Can you work these out from the model? Positions are in its coordinate system, mm. A direction names the side the tool comes from. Give positions to 0.01 mm unless a question says otherwise; leave off trailing zeros. Loops run counter-clockwise (first coordinate to the right, second up) from the corner with the lowest first, then second, coordinate; pieces in that order, holes last. Notation, with made-up numbers: (52, 65.5) -> (57, 65.5) arc R20 cw to (57, 86.5) -> close; hole circle Ø2 at (82, 75.5). An arc over 180 degrees is marked (long way). One line per question, with ' | ' between items.
from build123d import *

# Parameters (mm, degrees)
SKETCH_1_R      = 2.25
SKETCH_1_R_2    = 2.5
SKETCH_1_R_3    = 4
EXTRUDE_1_DEPTH = 2


with BuildPart() as part:
    # 草图1 → 凸台-拉伸1 (new body)
    with BuildSketch(Plane.XY):
        with BuildLine():
            Line((-97.333495067, -2.569668399), (0.921282848, -2.569581138))
            Line((0.921282848, -2.569581138), (99.176060763, -2.569468011))
            ThreePointArc((99.176060763, -2.569468011), (102.832215453, -3.990464351), (105.660516847, -6.708443184))
            ThreePointArc((105.660516847, -6.708443184), (128.420905518, 0.379743237), (105.718891057, 7.652721898))
            ThreePointArc((105.718891057, 7.652721898), (102.151642887, 4.54858247), (97.556982938, 3.430530125))
            Line((97.556982938, 3.430530125), (0.92127673, 3.430418862))
            Line((0.92127673, 3.430418862), (-95.714429479, 3.430333039))
            ThreePointArc((-95.714429479, 3.430333039), (-100.309091708, 4.548376014), (-103.876346209, 7.652508166))
            ThreePointArc((-103.876346209, 7.652508166), (-126.578345836, 0.379483205), (-103.81794271, -6.708656797))
            ThreePointArc((-103.81794271, -6.708656797), (-100.989646859, -3.990672195), (-97.333495067, -2.569668399))
        make_face()
        with Locations((-119.735572513, -5.226431967)):
            Circle(SKETCH_1_R, mode=Mode.SUBTRACT)
        with Locations((-121.081680504, 2.30686036)):
            Circle(SKETCH_1_R_2, mode=Mode.SUBTRACT)
        with Locations((-108.9521941, 5.556946446)):
            Circle(SKETCH_1_R_2, mode=Mode.SUBTRACT)
        with Locations((-112.202280186, -6.572539958)):
            Circle(SKETCH_1_R_2, mode=Mode.SUBTRACT)
        with Locations((-114.078604371, 0.43031673)):
            Circle(SKETCH_1_R_3, mode=Mode.SUBTRACT)
        with Locations((115.921163949, 0.430551269)):
            Circle(SKETCH_1_R_3, mode=Mode.SUBTRACT)
        with Locations((110.794757573, 5.556946446)):
            Circle(SKETCH_1_R_2, mode=Mode.SUBTRACT)
        with Locations((122.924243977, 2.30686036)):
            Circle(SKETCH_1_R_2, mode=Mode.SUBTRACT)
        with Locations((121.578135986, -5.226431967)):
            Circle(SKETCH_1_R, mode=Mode.SUBTRACT)
        with Locations((114.04484366, -6.572539958)):
            Circle(SKETCH_1_R_2, mode=Mode.SUBTRACT)
    extrude(amount=EXTRUDE_1_DEPTH)


solid = part.part
Q1. If we section it at B-B (x = 72): Write out the boundary of the cut face in (y, z).
Entries:
outline: (-2.57, 0) -> (3.43, 0) -> (3.43, 2) -> (-2.57, 2) -> close
Q2. For pin 1 Ø4.5 at (x, y) = (114.04, -6.57) entering from -Z; pin 2 Ø0.6 at (x, z) = (28.5, 1) entering from -Y; pin 3 Ø1 at (y, z) = (10, 1) entering from -X; pin 4 Ø1 at (x, z) = (30, 0.5) entering from +Y, each with a flat end and sliding along its axis, tell me the tip position at first contact or that it passes through.
Entries:
pin 1: through | pin 2: y = -2.57 | pin 3: x = -122.68 | pin 4: y = 3.43
Q3. If we mould it in two halves opening along X, with no side actions, what happens to faces 1 (the face through (116.43, -5.82, 0.99)), 2 (the face through (-1, 1, 0))? For each: pulls with the +X half, pulls with the -X half, needs draft (parallel to the pull), parting line crosses it, or undercut.
Entries:
face 1: undercut | face 2: needs draft
Q4. If I drill on probe 1 along X at (y, z) = (-5.5, 0.2); probe 2 along X at (y, z) = (-3.25, 0.8); probe 3 along X at (y, z) = (7.25, 0.8), over which ranges is the centre line in solid material (lowest first)? Write a range as from..to.
Entries:
probe 1: -125.08..-121.97, -117.5..-114.46, -109.94..-102.83, 104.67..111.79, 116.3..119.34, 123.81..126.92 | probe 2: -126.02..-120.81, -118.66..-115.65, -112.51..-99.6, 101.44..114.35, 117.49..120.5, 122.65..127.87 | probe 3: -124.55..-110.79, -107.11..-103.58, 105.42..108.96, 112.63..126.4
Q5. On a 3-axis mill with a long thin cutter (end or side, diameter ignored), from which of +Z, -Z, +X, -X, +Y, -Y can I reach the whole of each face in a straight line? I mean faces 3 (the face through (102.21, 4.58, 0.99)), 4 (the face through (-101.036, -4.021, 0.986)), 5 (the face through (119.33, -5.13, 0.99)). Say none if no direction works.
Entries:
face 3: +Z, -Z, +Y | face 4: +Z, -Z, -Y | face 5: +Z, -Z
Q6. If we section it at A-A (z = 1.05): State how many separate pieces and enclosed holes the cut face has, plus the area to 3 significant figures.
Entries:
separate pieces: 1 | enclosed holes: 10 | area: 1,980 mm²
